The model under review builds one solid part; all positions refer to its coordinate system, in mm. Coordinates: 2 decimals unless noted, no trailing zeros. Order: outer loops, then holes, each group sorted by start corner. A loop starts at its lowest first (then second) coordinate and runs counter-clockwise, first axis right, second up. Notation, with made-up numbers: M 54.25,25.5 L 80.25,25.5 A18 ccw 80.25,59.5 Z; hole C 48.25,75.5 d5. An arc over 180 degrees is marked long. One line per item, written item: value.
Autodesk Inventor part; units mm, degrees
ref_plane "YZ Plane" through (0, 0, 0) normal (1, 0, 0) x (0, 1, 0)
ref_plane "XZ Plane" through (0, 0, 0) normal (0, 1, 0) x (-1, 0, 0)
ref_plane "XY Plane" through (0, 0, 0) normal (0, 0, 1) x (1, 0, 0)
sketch "Sketch1" plane through (0, 0, 0) normal (0, 1, 0) x (-1, 0, 0)
  arc A0 (0, 5.4545) -> (0, -5.4545) centre (0, 0) ccw
  arc A1 (170, -5.4545) -> (170, 5.4545) centre (170, 0) ccw
  line L0 (0, 5.4545) -> (170, 5.4545)
  line L1 (170, -5.4545) -> (0, -5.4545)
  dimension "d0" = 10.909
  dimension "d1" = 10.909
  dimension "d2" = 170
extrude "Extrusion1" add sketch "Sketch1" along normal blind 1.7
sketch "Sketch2" plane through (0, 1.7, 0) normal (0, 1, 0) x (1, 0, 0)
  arc A0 (0, -5.4545) -> (0, 5.4545) centre (0, 0) ccw
  arc A1 (-170, 5.4545) -> (-170, -5.4545) centre (-170, 0) ccw
  circle A2 centre (0, 0) radius 1.5
  circle A3 centre (-170, 0) radius 1.5
  dimension "d5" = 3
  dimension "d6" = 3
extrude "Extrusion2" cut sketch "Sketch2" against normal blind 1.7
equation "\"BendRadius\" = Thickness"
equation "\"BendReliefWidth\" = Thickness"
equation "\"BendReliefDepth\" = 0.5 * Thickness"
equation "\"CornerReliefSize\" = 4 * Thickness"
equation "\"MinimumRemnant\" = 2 * Thickness"
equation "\"TransitionRadius\" = BendRadius"
equation "\"JacobiRadiusSize\" = BendRadius"
equation "\"GapSize\" = Thickness"
properties part number "A1P2"
(1) Mouldability with a two-part tool opening along X and no side actions: class faces 1 (the cylindrical face through (-168.614, 0.862, 0.575)), 2 (the flat face through (-84, 0, 0)), 3 (the cylindrical face through (-175.453, 0.838, 0.12)) as +X half, -X half, draft (parallel to the pull), parting line (faces both ways), or undercut.
Geometry results:
face 1: undercut
face 2: draft
face 3: -X half
(2) We need section B-B, the plane y = 1.35. State the section outline as (x, z) points, plus the area to 3 significant figures.
Geometry results:
outline: M -170,-5.45 L 0,-5.45 A5.45 ccw 0,5.45 L -170,5.45 A5.45 ccw Z; hole C -170,0 d3; hole C 0,0 d3
area: 1,930 mm2
(3) We need section A-A, the plane z = 0. State the section outline as (x, y) points, plus the area to 3 significant figures.
Geometry results:
outline: M -175.45,0 L -171.5,0 L -171.5,1.7 L -175.45,1.7 Z; M -168.5,0 L -1.5,0 L -1.5,1.7 L -168.5,1.7 Z; M 1.5,0 L 5.45,0 L 5.45,1.7 L 1.5,1.7 Z
area: 297 mm2
(4) For L1, parallel to X at y = 0.9, z = 0; L2, parallel to Z at x = 0, y = 1.35; L3, parallel to X at y = 0.7, z = 1, list the stretches that pass through material, from the lowest coordinate up.
Geometry results:
L1: x = -175.45 to -171.5, -168.5 to -1.5, 1.5 to 5.45
L2: z = -5.45 to -1.5, 1.5 to 5.45
L3: x = -175.36 to -171.12, -168.88 to -1.12, 1.12 to 5.36
